from build123d import *

# Parameters (mm, degrees)
F1_DEPTH = 40
F3_D     = 14
F3_DEPTH = 3
F3_TIP   = 4.2060243332
F5_D     = 12


with BuildPart() as f1:
    # F0 (on Top) → F1 (new body)
    with BuildSketch(Plane.XY):
        with BuildLine():
            Line((-12.5, -20), (12.5, -20))
            ThreePointArc((12.5, -20), (17.8033008589, -17.8033008589), (20, -12.5))
            Line((20, -12.5), (20, 12.5))
            ThreePointArc((20, 12.5), (17.8033008589, 17.8033008589), (12.5, 20))
            Line((12.5, 20), (-12.5, 20))
            ThreePointArc((-12.5, 20), (-17.8033008589, 17.8033008589), (-20, 12.5))
            Line((-20, 12.5), (-20, -12.5))
            ThreePointArc((-20, -12.5), (-17.8033008589, -17.8033008589), (-12.5, -20))
        make_face()
        with BuildLine():
            ThreePointArc((-12.5, -17), (-15.6819805153, -15.6819805153), (-17, -12.5))
            Line((-17, -12.5), (-17, 12.5))
            ThreePointArc((-17, 12.5), (-15.6819805153, 15.6819805153), (-12.5, 17))
            Line((-12.5, 17), (12.5, 17))
            ThreePointArc((12.5, 17), (15.6819805153, 15.6819805153), (17, 12.5))
            Line((17, 12.5), (17, -12.5))
            ThreePointArc((17, -12.5), (15.6819805153, -15.6819805153), (12.5, -17))
            Line((12.5, -17), (-12.5, -17))
        make_face(mode=Mode.SUBTRACT)
    extrude(amount=F1_DEPTH)

    # F3
    with Locations(Plane.XZ.offset(20)):
        with Locations((-3.5, 30)):
            Hole(F3_D / 2, depth=F3_DEPTH)
            with Locations((0, 0, -(F3_DEPTH + F3_TIP / 2))):  # 118° drill point
                Cone(0, F3_D / 2, F3_TIP, mode=Mode.SUBTRACT)

    # F5 (through all)
    with Locations(Plane.YZ.offset(20)):
        with Locations((0, 10)):
            Hole(F5_D / 2)


solid = f1.part
Source: CAD feature listing. Evaluate the final solid. Frame: model axes, mm. A direction names the side the tool comes from. Round coordinates to 2 decimals unless told otherwise and drop trailing zeros. Loops run counter-clockwise (first coordinate to the right, second up) from the corner with the lowest first, then second, coordinate; pieces in that order, holes last.
Q1. Access query for faces 1 (the face through (-17.861, -17.745, 19.72)), 2 (the face through (-1.983, -18.479, 23.166)), 3 (the face through (15.647, 15.717, 19.72)). Directions: +Z, -Z, +X, -X, +Y, -Y. A direction counts if a zero-diameter tool reaches every point of the face in a straight line with its end or side. Return the directions, or none.
Q2. Section C-C, the plane y = -7. Return loops of the section in (x, z), plus the area to 3 significant figures.
Q3. Section A-A, the plane x = -3.5. Return loops of the section in (y, z), plus the area to 3 significant figures.
Q4. Section B-B, the plane z = 10. Return loops of the section in (x, y).
Q5. First-contact query: P1, Ø7.5, axis at x = -4, z = 27.5, coming from the -Y side; P2, Ø1.5, axis at x = -13.5, z = 26, coming from the -Y side. Flat tips, straight axial feed; report the tip coordinate or a pass-through.
Q6. Ray query, line 1 (Y direction, x = 12, z = 3.5); line 2 (Z direction, x = 19, y = 0). Return the intervals inside material, ascending.
Q7. Mould query, pull axis Z, two halves, no side actions, for faces 4 (the face through (0, -17, 20)), 5 (the face through (-0.3, -17.5, 0)), 6 (the face through (18.479, 1.301, 4.143)). Classes: pulls with the +Z half, pulls with the -Z half, needs draft (parallel to the pull), parting line crosses it, or undercut.
Solutions:
1. face 1: +Z, -Z, -X, -Y
1. face 2: -Y
1. face 3: +Z, -Z
2. outline: (-20, 0) - (-17, 0) - (-17, 40) - (-20, 40) - close; (17, 0) - (20, 0) - (20, 40) - (17, 40) - close
2. area: 240 mm2
3. outline: (-20, 0) - (-17, 0) - (-17, 23) - (-20, 23) - close; (-20, 37) - (-17, 37) - (-17, 40) - (-20, 40) - close; (17, 0) - (20, 0) - (20, 40) - (17, 40) - close
3. area: 198 mm2
4. outline: (-20, -12.5) arc R7.5 ccw to (-12.5, -20) - (12.5, -20) arc R7.5 ccw to (20, -12.5) - (20, -6) - (17, -6) - (17, -12.5) arc R4.5 cw to (12.5, -17) - (-12.5, -17) arc R4.5 cw to (-17, -12.5) - (-17, -6) - (-20, -6) - close; (-20, 6) - (-17, 6) - (-17, 12.5) arc R4.5 cw to (-12.5, 17) - (12.5, 17) arc R4.5 cw to (17, 12.5) - (17, 6) - (20, 6) - (20, 12.5) arc R7.5 ccw to (12.5, 20) - (-12.5, 20) arc R7.5 ccw to (-20, 12.5) - close
5. P1: stops at y = 17
5. P2: stops at y = -20
6. line 1: y = -20 to -17, 17 to 20
6. line 2: z = 0 to 4, 16 to 40
7. face 4: needs draft
7. face 5: pulls with the -Z half
7. face 6: undercut
